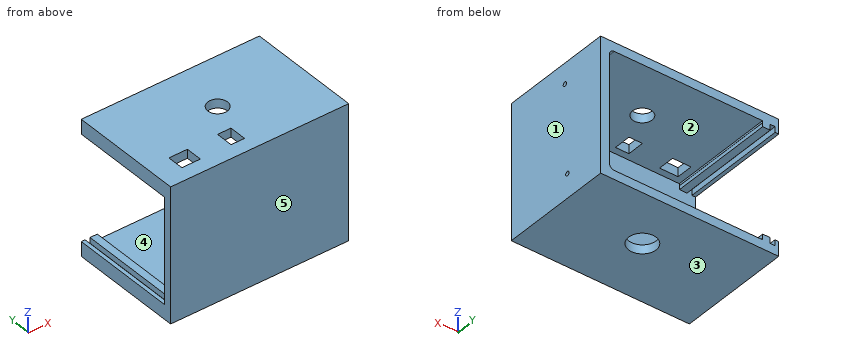
Autodesk Inventor part; units mm, degrees
ref_plane "YZ Plane" through (0, 0, 0) normal (1, 0, 0) x (0, 1, 0)
ref_plane "XZ Plane" through (0, 0, 0) normal (0, 1, 0) x (-1, 0, 0)
ref_plane "XY Plane" through (0, 0, 0) normal (0, 0, 1) x (1, 0, 0)
sketch "Sketch1" plane through (0, 0, 0) normal (0, 1, 0) x (-1, 0, 0)
  line L0 (50.8, 37.719) -> (-50.8, 37.719)
  line L1 (-50.8, 37.719) -> (-50.8, -37.719)
  line L2 (-50.8, -37.719) -> (50.8, -37.719)
  line L3 (50.8, -37.719) -> (50.8, 37.719)
  line L4 (50.8, 37.719) -> (-50.8, -37.719) construction
  line L5 (-50.8, 37.719) -> (50.8, -37.719) construction
  line L6 (56.515, 43.434) -> (-56.515, 43.434)
  line L7 (-56.515, 43.434) -> (-56.515, -43.434)
  line L8 (-56.515, -43.434) -> (56.515, -43.434)
  line L9 (56.515, -43.434) -> (56.515, 43.434)
  line L10 (56.515, 43.434) -> (-56.515, -43.434) construction
  line L11 (-56.515, 43.434) -> (56.515, -43.434) construction
  point P0 (0, 0)
  dimension "d0" = 101.6
  dimension "d1" = 75.438
  dimension "d2" = 113.03
  dimension "d3" = 86.868
extrude "Extrusion1" add sketch "Sketch1" along normal blind 68.58
sketch "Sketch2" plane through (0, 0, 0) normal (0, -1, 0) x (1, 0, 0)
  line L0 (-50.8, 37.719) -> (50.8, 37.719)
  line L1 (-50.8, 37.719) -> (-41.656, 37.719)
  line L2 (-50.8, 37.719) -> (-50.8, -37.719)
  line L3 (-41.656, 37.719) -> (-50.8, 37.719)
  line L4 (-50.8, 37.719) -> (-41.656, 37.719)
  point P0 (0, 0)
  dimension "d6" = 9.144
sketch "Sketch3" plane through (-56.515, 0, 43.434) normal (0, 0, 1) x (1, 0, 0)
  line L0 (12.3133, 0) -> (12.3133, 10.668)
  line L1 (12.3133, 10.668) -> (12.3133, 14.986)
  line L2 (12.3133, 14.986) -> (24.3021, 14.986)
  line L3 (24.3021, 14.986) -> (24.3021, 4.318)
  line L4 (24.3021, 4.318) -> (12.3133, 4.318)
  line L5 (0, 0) -> (113.03, 0)
  line L6 (24.3021, 4.318) -> (44.2157, 4.318)
  line L7 (44.2157, 4.318) -> (44.2157, 15.494)
  line L8 (44.2157, 15.494) -> (52.9279, 15.494)
  line L9 (52.9279, 15.494) -> (52.9279, 4.318)
  line L10 (52.9279, 4.318) -> (44.2157, 4.318)
  point P0 (56.515, 0)
  dimension "d7" = 10.668
  dimension "d8" = 4.318
  dimension "d9" = 11.9888
  dimension "d10" = 10.668
  dimension "d11" = 19.9136
  dimension "d12" = 11.176
  dimension "d13" = 8.7122
extrude "Extrusion2" cut sketch "Sketch3" against normal blind 68.58
sketch "Sketch4" plane through (50.8, 0, 37.719) normal (-1, 0, 0) x (0, 0, 1)
  line L0 (0, 0) -> (-75.438, 0)
  line L1 (-75.438, 0) -> (-34.29, 0)
  line L2 (-34.29, 0) -> (-75.438, 0)
  line L3 (-75.438, 0) -> (-75.438, 68.58)
  line L4 (-75.438, 0) -> (-75.438, 41.148)
  line L5 (-75.438, 41.148) -> (-65.532, 41.148)
  line L6 (-65.532, 41.148) -> (-75.438, 41.148)
  line L7 (0, 0) -> (0, 68.58)
  line L8 (0, 68.58) -> (0, 39.116)
  line L9 (0, 39.116) -> (0, 46.736)
  line L10 (0, 46.736) -> (0, 39.116)
  line L11 (0, 39.116) -> (-7.62, 39.116)
  line L12 (-7.62, 39.116) -> (0, 39.116)
  circle A0 centre (-7.62, 39.116) radius 1.397
  circle A1 centre (-65.532, 41.148) radius 1.397
  point P0 (-37.719, 0)
  dimension "d16" = 41.148
  dimension "d17" = 41.148
  dimension "d18" = 9.906
  dimension "d19" = 29.464
  dimension "d20" = 7.62
  dimension "d21" = 7.62
  dimension "d22" = 2.794
  dimension "d23" = 2.794
extrude "Extrusion3" cut sketch "Sketch4" against normal blind 68.58
sketch "Sketch5" plane through (-56.515, 0, 43.434) normal (0, 0, 1) x (1, 0, 0)
  point P0 (56.515, 0)
sketch "Sketch6" plane through (-56.515, 0, 43.434) normal (0, 0, 1) x (1, 0, 0)
  line L0 (0, 0) -> (0, 68.58)
  line L1 (113.03, 0) -> (113.03, 68.58)
  line L2 (0, 68.58) -> (113.03, 0)
  line L3 (113.03, 0) -> (0, 68.58)
  line L4 (0, 68.58) -> (113.03, 68.58)
  line L5 (113.03, 68.58) -> (5.08, 0)
  line L6 (5.08, 0) -> (113.03, 68.58)
  circle A0 centre (59.055, 34.29) radius 6.35
  point P0 (56.515, 0)
  dimension "d26" = 12.7
extrude "Extrusion4" cut sketch "Sketch6" against normal blind 109.855 contours A0 L5 L2 | L2 L5 A0 | L5 L2 A0 | L5 A0 L2
sketch "Sketch7" plane through (0, 0, 0) normal (0, -1, 0) x (1, 0, 0)
  line L0 (-56.515, 43.434) -> (56.515, 43.434)
  line L1 (56.515, 43.434) -> (56.515, -43.434)
  line L2 (-56.515, 43.434) -> (56.515, 43.434)
  line L3 (56.515, 43.434) -> (56.515, -43.434)
  line L4 (56.515, -43.434) -> (-56.515, -43.434)
  line L5 (-56.515, -43.434) -> (-56.515, 43.434)
  point P0 (0, 0)
extrude "Extrusion5" add sketch "Sketch7" along normal blind 5.08
sketch "Sketch9" plane through (0, 68.58, 0) normal (0, 1, 0) x (1, 0, 0)
  point P0 (0, 0)
sketch "Sketch10" plane through (50.8, 68.58, -37.719) normal (-1, 0, 0) x (0, 0, 1)
  circle A0 centre (67.818, -29.464) radius 1.397
  circle A1 centre (67.818, -29.464) radius 3.302
  circle A2 centre (9.906, -27.432) radius 1.397
  circle A3 centre (9.906, -27.432) radius 3.302
  point P0 (37.719, -68.58)
  dimension "d36" = 6.604
  dimension "d37" = 6.604
extrude "Extrusion7" add sketch "Sketch10" along normal blind 12.7
sketch "Sketch11" plane through (-56.515, 68.58, -43.434) normal (-1, 0, 0) x (0, 0, 1)
  line L0 (5.715, -68.58) -> (5.715, 0)
  line L1 (81.153, -68.58) -> (81.153, 0)
  line L2 (5.715, 0) -> (81.153, 0)
  line L3 (81.153, 0) -> (81.153, -68.58)
  line L4 (81.153, -68.58) -> (5.715, -68.58)
  line L5 (5.715, -68.58) -> (5.715, 0)
  point P0 (43.434, -68.58)
extrude "Extrusion8" cut sketch "Sketch11" against normal blind 12.7
fillet "Fillet2" radius 3.175 3 edges at (50.8, 34.29, -37.719) (50.8, 0, 0) (50.8, 34.29, 37.719)
sketch "Sketch12" plane through (56.515, 68.58, -43.434) normal (0, 0, -1) x (-1, 0, 0)
  circle A0 centre (53.975, -34.29) radius 4.445
  circle A1 centre (53.975, -34.29) radius 8.89
  circle A2 centre (53.975, -34.29) radius 6.35
  point P0 (56.515, -68.58)
  dimension "d43" = 8.89
  dimension "d44" = 17.78
extrude "Extrusion9" cut sketch "Sketch12" against normal blind 12.7 contours A1
sketch "Sketch13" plane through (0, 0, 0) normal (0, 1, 0) x (1, 0, 0)
  line L0 (-56.515, 37.719) -> (47.625, 37.719)
  line L1 (-50.7189, 37.719) -> (-49.9627, 37.719)
  line L2 (-49.9627, 37.719) -> (-49.9627, 36.449)
  line L3 (-49.9627, 36.449) -> (-50.7189, 36.449)
  line L4 (-50.7189, 36.449) -> (-50.7189, 37.719)
  line L5 (-56.515, -37.719) -> (47.625, -37.719)
  line L6 (-50.7189, -37.719) -> (-49.9627, -37.719)
  line L7 (-49.9627, -37.719) -> (-49.9627, -36.449)
  line L8 (-49.9627, -36.449) -> (-50.7189, -36.449)
  line L9 (-50.7189, -36.449) -> (-50.7189, -37.719)
  point P0 (0, 0)
  dimension "d47" = 1.27
  dimension "d48" = 1.27
extrude "Extrusion10" add sketch "Sketch13" along normal blind 68.58
sketch "Sketch14" plane through (-56.515, -5.08, -43.434) normal (-1, 0, 0) x (0, 0, 1)
  point P0 (43.434, 5.08)
sketch "Sketch15" plane through (-56.515, -5.08, -43.434) normal (-1, 0, 0) x (0, 0, 1)
  line L0 (0, 73.66) -> (5.715, 73.66)
  line L1 (86.868, 0) -> (0, 0)
  line L2 (0, 73.66) -> (4.5789, 73.66)
  line L3 (4.5789, 73.66) -> (4.5789, 0)
  line L4 (4.5789, 0) -> (0, 0)
  line L5 (0, 0) -> (0, 73.66)
  line L6 (81.153, 73.66) -> (86.868, 73.66)
  line L7 (86.868, 73.66) -> (77.4615, 73.66)
  line L8 (77.4615, 73.66) -> (77.4615, 0)
  line L9 (77.4615, 0) -> (86.868, 0)
  line L10 (86.868, 0) -> (86.868, 73.66)
  line L11 (4.5789, 0) -> (77.4615, 0)
  line L12 (77.4615, 0) -> (77.4615, 5.08)
  line L13 (77.4615, 5.08) -> (4.5789, 5.08)
  line L14 (4.5789, 5.08) -> (4.5789, 0)
  point P0 (43.434, 5.08)
extrude "Extrusion11" add sketch "Sketch15" along normal blind 0.762
sketch "Sketch16" plane through (-57.277, -5.08, -43.434) normal (-1, 0, 0) x (0, 0, 1)
  line L0 (0, 0) -> (86.868, 0)
  line L1 (0, 73.66) -> (4.5551, 73.66)
  line L2 (4.5551, 73.66) -> (4.5551, 0)
  line L3 (4.5551, 0) -> (0, 0)
  line L4 (0, 0) -> (0, 73.66)
  line L5 (86.868, 73.66) -> (77.4615, 73.66)
  line L6 (86.868, 0) -> (86.868, 73.66)
  line L7 (77.4615, 73.66) -> (86.868, 73.66)
  line L8 (86.868, 73.66) -> (86.868, 0)
  line L9 (86.868, 0) -> (77.4615, 0)
  line L10 (77.4615, 0) -> (77.4615, 73.66)
  line L11 (79.883, 5.08) -> (81.153, 5.08)
  line L12 (79.883, 5.08) -> (4.5551, 5.08)
  line L13 (4.5551, 5.08) -> (4.5551, 0)
  line L14 (4.5551, 0) -> (79.883, 0)
  line L15 (79.883, 0) -> (79.883, 5.08)
  point P0 (43.434, 5.08)
extrude "Extrusion12" add sketch "Sketch16" along normal blind 1.5875
sketch "Sketch17" plane through (-49.9627, 0, 36.449) normal (1, 0, 0) x (0, 0, -1)
  line L0 (-1.27, 68.58) -> (0, 68.58)
  line L1 (0, 68.58) -> (-1.27, 68.58)
  line L2 (-1.27, 68.58) -> (-1.27, 0)
  line L3 (-1.27, 0) -> (0, 0)
  line L4 (0, 0) -> (0, 68.58)
  line L5 (74.168, 0) -> (72.898, 0)
  line L6 (72.898, 0) -> (72.898, 68.58)
  line L7 (74.168, 0) -> (72.898, 0)
  line L8 (72.898, 0) -> (72.898, 68.58)
  line L9 (72.898, 68.58) -> (74.168, 68.58)
  line L10 (74.168, 68.58) -> (74.168, 0)
  point P0 (36.449, 0)
extrude "Extrusion13" add sketch "Sketch17" along normal blind 1.5875
sketch "Sketch18" plane through (-50.7189, 0, -36.449) normal (-1, 0, 0) x (0, 0, 1)
  point P0 (36.449, 0)
sketch "Sketch19" plane through (-57.277, 0, -38.8789) normal (0, 0, 1) x (1, 0, 0)
  line L0 (-1.5875, 68.58) -> (-1.5875, -5.08)
  line L1 (-1.5875, 68.58) -> (0.8838, 68.58)
  line L2 (0.8838, 68.58) -> (0.8838, 0)
  line L3 (0.8838, 0) -> (-1.5875, 0)
  line L4 (-1.5875, 0) -> (-1.5875, 68.58)
  point P0 (57.277, 0)
extrude "Extrusion14" add sketch "Sketch19" along normal blind 4.826
sketch "Sketch20" plane through (0, 68.58, 0) normal (0, 1, 0) x (1, 0, 0)
  point P0 (0, 0)
sketch "Sketch21" plane through (0, 0, 0) normal (0, 1, 0) x (1, 0, 0)
  line L0 (-56.515, -37.719) -> (-56.515, -34.0275)
  line L1 (-56.515, -37.719) -> (-53.34, -37.719)
  line L2 (-50.7189, -37.719) -> (-56.515, -37.719)
  line L3 (-53.34, -37.719) -> (-56.515, -37.719)
  line L4 (-56.3932, 37.719) -> (-56.3932, 34.0529)
  line L5 (-56.3932, 37.719) -> (-53.2182, 37.719)
  line L6 (-56.3932, 37.719) -> (-50.7189, 37.719)
  line L7 (-53.2182, 37.719) -> (-56.3932, 37.719)
  line L8 (-53.2182, 37.719) -> (-48.4756, 37.719)
  line L9 (-48.4756, 37.719) -> (-48.4756, 34.0529)
  line L10 (-48.4756, 34.0529) -> (-53.2182, 34.0529)
  line L11 (-53.2182, 34.0529) -> (-53.2182, 37.719)
  line L12 (-53.34, -37.719) -> (-48.4756, -37.719)
  line L13 (-48.4756, -37.719) -> (-48.4756, -34.0275)
  line L14 (-48.4756, -34.0275) -> (-53.34, -34.0275)
  line L15 (-53.34, -34.0275) -> (-53.34, -37.719)
  point P0 (0, 0)
  dimension "d59" = 3.175
  dimension "d60" = 3.175
extrude "Extrusion15" add sketch "Sketch21" along normal blind 68.58
properties part number "Boxpt1"
Input: part model. Units: mm. Frame: model coordinates. Face numbers are marked on the shaded views. A direction names the side the tool comes from. Give positions to 0.01 mm unless a question says otherwise; leave off trailing zeros. Write each loop counter-clockwise with the first axis right and the second up, starting at its lowest first coordinate (ties: lowest second). Pieces come first, ordered by that corner, then holes. Notation, with made-up numbers: (-38.5, 45) - (13.5, 45) arc R18 cw to (13.5, 50) - close; hole circle Ø2 at (36, 39.25). An arc over 180 degrees is marked (long way). Write item = value, one per line. Start each with the question number.
1) Cut plane A-A (x = -9.5). Return loops of the section in (y, z).
2) Cut plane B-B (y = 34.29). Give the number of separate pieces and of enclosed holes in the cut face, and give its area (3 significant figures).
3) Pin query (flat end, axial travel): pin 1 (1.5 mm diameter, centred on y = 44.5, z = 1.5, fed in from -X); pin 2 (2.5 mm diameter, centred on y = 39.116, z = 30.099, fed in from -X); pin 3 (14.5 mm diameter, centred on x = 2.54, y = 34.29, fed in from -Z); pin 4 (2 mm diameter, centred on x = 20, z = -7.5, fed in from +Y). Return the tip coordinate at first contact, or that it passes through.
4) Cut plane C-C (x = 2.54). Return loops of the section in (y, z), and give its area (3 significant figures).
5) Reachability of the marked faces 4 and 5 from +Z, -Z, +X, -X, +Y, -Y: full face, straight path, thin tool, end or side. Return the list, or none.
6) Material intervals for L1, parallel to Z at x = 42.5, y = 12.5; L2, parallel to Y at x = 2, z = 39; L3, parallel to X at y = 26, z = 36.5 (1 decimal), sorted ascending. Write a range as [from, to].
7) Draft query along X for the marked faces 1, 2 and 3. Return one class per face: pulls with the +X half, pulls with the -X half, needs draft (parallel to the pull), parting line crosses it, or undercut.
Answers follow:
q1.outline = (-5.08, -43.43) - (68.58, -43.43) - (68.58, -37.72) - (0, -37.72) - (0, 37.72) - (4.32, 37.72) - (4.32, 43.43) - (-5.08, 43.43) - close; (15.49, 37.72) - (68.58, 37.72) - (68.58, 43.43) - (15.49, 43.43) - close
q2.separate_pieces = 3
q2.enclosed_holes = 0
q2.area = 1,630 mm^2
q3.pin_1 = 50.8
q3.pin_2 = through
q3.pin_3 = 37.72
q3.pin_4 = 0
q4.outline = (-5.08, -43.43) - (25.4, -43.43) - (25.4, -37.72) - (0, -37.72) - (0, 37.72) - (27.94, 37.72) - (27.94, 43.43) - (-5.08, 43.43) - close; (40.64, 37.72) - (68.58, 37.72) - (68.58, 43.43) - (40.64, 43.43) - close; (43.18, -43.43) - (68.58, -43.43) - (68.58, -37.72) - (43.18, -37.72) - close
q4.area = 1,050 mm^2
q5.face_4 = +Y
q5.face_5 = +Z, -Z, +X, -X, -Y
q6.L1 = [-43.43, -37.72], [37.72, 43.43]
q6.L2 = [-5.08, 27.96], [40.62, 68.58]
q6.L3 = [-58.9, -56.5], [-53.3, -48.4], [50.1, 56.5]
q7.face_1 = pulls with the +X half
q7.face_2 = undercut
q7.face_3 = needs draft
